Job drawing, mm, ordinate dimensions from the low corner. One solid piece. Give positions to 0.01 mm unless a question says otherwise; leave off trailing zeros. Order: outer loops, then holes, each group sorted by start corner. A loop starts at its lowest first (then second) coordinate and runs counter-clockwise, first axis right, second up. Notation, with made-up numbers: M 78.5,40.25 L 85.5,40.25 A24 ccw 85.5,52.25 Z; hole C -4.5,59.5 d10. An arc over 180 degrees is marked long. Use CSV: the item, a comma, the result in double quotes. Start each with the question number.
Item 1: Band-saw the part on D-D on x = 197. Write the cut outline in (y, z).
Item 2: Pin check, flat tips, straight feed: P1, Ø3, axis at y = 2.5, z = 113.5, coming from the -X side; P2, Ø2, axis at y = 4, z = 55.5, coming from the +X side; P3, Ø1.9, axis at x = 18.5, y = 4.5, coming from the +Z side. Stop position of each tip, or through.
Item 3: Band-saw the part on A-A on y = 1.5. Write the cut outline in (x, z).
Item 4: Wall check: line 1 along Z through (x, y) = (76.2, 3.5); line 2 along Z through (x, y) = (169, 1.75); line 3 along X through (y, z) = (4.25, 95). Give the ranges that are in metal, low to high.
Item 5: Band-saw the part on B-B on x = 76.2. Write the cut outline in (y, z), plus the area to 3 significant figures.
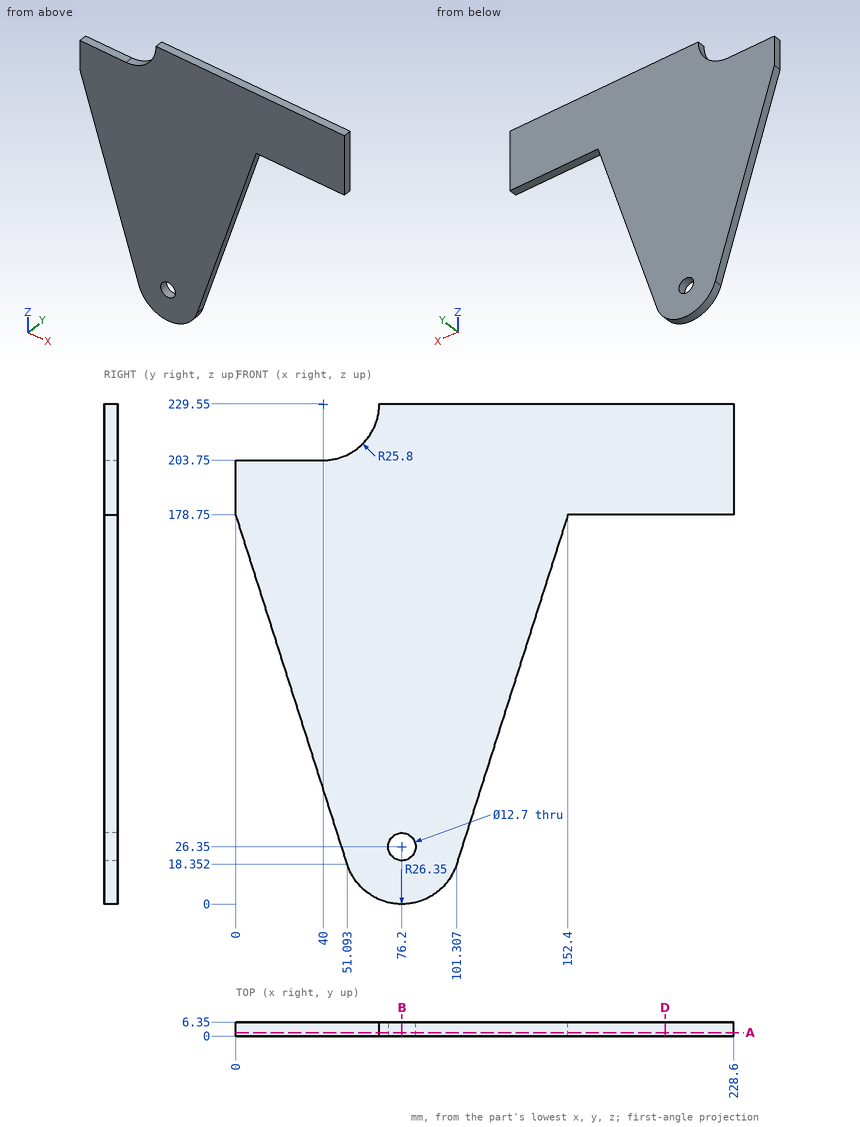
Model answer:
1,outline,"M 0,178.75 L 6.35,178.75 L 6.35,229.55 L 0,229.55 Z"
2,P1,"stops at x = 20.31"
2,P2,"stops at x = 113.46"
2,P3,"stops at z = 203.75"
3,outline,"M 0,178.75 L 51.09,18.35 A26.35 ccw 101.31,18.35 L 152.4,178.75 L 228.6,178.75 L 228.6,229.55 L 65.8,229.55 A25.8 cw 40,203.75 L 0,203.75 Z; hole C 76.2,26.35 d12.7"
4,line 1,"z = 0 to 20, 32.7 to 229.55"
4,line 2,"z = 178.75 to 229.55"
4,line 3,"x = 26.68 to 125.72"
5,outline,"M 0,0 L 6.35,0 L 6.35,20 L 0,20 Z; M 0,32.7 L 6.35,32.7 L 6.35,229.55 L 0,229.55 Z"
5,area,"1,380 mm^2"
